from build123d import *

# Parameters (mm, degrees)
F0_W     = 762
F0_H     = 203.2
F1_DEPTH = 6.35
F2_W     = 127
F2_H     = 63.5
F3_DEPTH = 25.4
F4_W     = 127
F4_H     = 63.5
F5_DEPTH = 25.4
F6_W     = 127
F6_H     = 63.5
F7_DEPTH = 25.4
F8_W     = 127
F8_H     = 63.5
F9_DEPTH = 25.4
F10_R    = 6.34999


# Not quite as in the source:
# - a fillet or chamfer is up to 0.001 mm smaller than in the source, because OpenCascade refuses the exact size


with BuildPart() as f1:
    # F0 (on Top) → F1 (new body)
    with BuildSketch(Plane.XY):
        Rectangle(F0_W, F0_H)
    extrude(amount=F1_DEPTH)

    # F2 (on face) → F3 (cut)
    with BuildSketch(Plane.XY.offset(6.35)):
        with Locations((317.5, 69.85)):
            Rectangle(F2_W, F2_H)
    extrude(amount=-F3_DEPTH, mode=Mode.SUBTRACT)

    # F4 (on face) → F5 (cut)
    with BuildSketch(Plane.XY.offset(6.35)):
        with Locations((317.5, -69.85)):
            Rectangle(F4_W, F4_H)
    extrude(amount=-F5_DEPTH, mode=Mode.SUBTRACT)

    # F6 (on face) → F7 (cut)
    with BuildSketch(Plane.XY.offset(6.35)):
        with Locations((-317.5, 69.85)):
            Rectangle(F6_W, F6_H)
    extrude(amount=-F7_DEPTH, mode=Mode.SUBTRACT)

    # F8 (on face) → F9 (cut)
    with BuildSketch(Plane.XY.offset(6.35)):
        with Locations((-317.5, -69.85)):
            Rectangle(F8_W, F8_H)
    extrude(amount=-F9_DEPTH, mode=Mode.SUBTRACT)

    # F10 (radius 6.35 in the source; OpenCascade refuses exactly that, so slightly less here)
    f10_edges = [f1.edges().sort_by_distance(p)[0] for p in [
        (-317.5, 38.1, 6.35),
        (-254, 69.85, 6.35),
        (0, 101.6, 6.35),
        (254, 69.85, 6.35),
        (317.5, 38.1, 6.35),
        (381, 0, 6.35),
        (317.5, -38.1, 6.35),
        (254, -69.85, 6.35),
        (0, -101.6, 6.35),
        (-254, -69.85, 6.35),
        (-317.5, -38.1, 6.35),
        (-381, 0, 6.35),
    ]]
    fillet(f10_edges, radius=F10_R)


solid = f1.part
Could you check a few things on this model? Use its own coordinates, in mm. Give positions to 0.01 mm unless a question says otherwise; leave off trailing zeros. Order: outer loops, then holes, each group sorted by start corner. A loop starts at its lowest first (then second) coordinate and runs counter-clockwise, first axis right, second up. Notation, with made-up numbers: (-12.75, 2.5) - (-0.75, 2.5) arc R25 cw to (-0.75, 26.5) - close; hole circle Ø7 at (52, 26). An arc over 180 degrees is marked (long way). Return JSON: item names as keys, results as strings. Group by question number.
Q1. Please list where these lines run through material, in increasing order: line 1 along Y through (x, z) = (214, 0.5); line 2 along X through (y, z) = (-93, 0.5); line 3 along Y through (x, z) = (47.5, 2). Write a range as [from, to].
Q2. Suppose I cut it at C-C, the plane z = 3.75. Please give me the cut outline in (x, y).
Q3. Will these pins go through, and if not, where does the flat tip stop? pin 1 Ø3 at (y, z) = (-46, 1.5) entering from +X; pin 2 Ø1 at (y, z) = (-33, 2.5) entering from -X.
Resolved:
{
 "1": {"line 1": "y = [-101.58, 101.58]", "line 2": "x = [-253.98, 253.98]", "line 3": "y = [-101.28, 101.28]"},
 "2": {"outline": "(-379.77, -36.87) - (-252.77, -36.87) - (-252.77, -100.37) - (252.77, -100.37) - (252.77, -36.87) - (379.77, -36.87) - (379.77, 36.87) - (252.77, 36.87) - (252.77, 100.37) - (-252.77, 100.37) - (-252.77, 36.87) - (-379.77, 36.87) - close"},
 "3": {"pin 1": "stops at x = 254", "pin 2": "stops at x = -380.68"}
}
